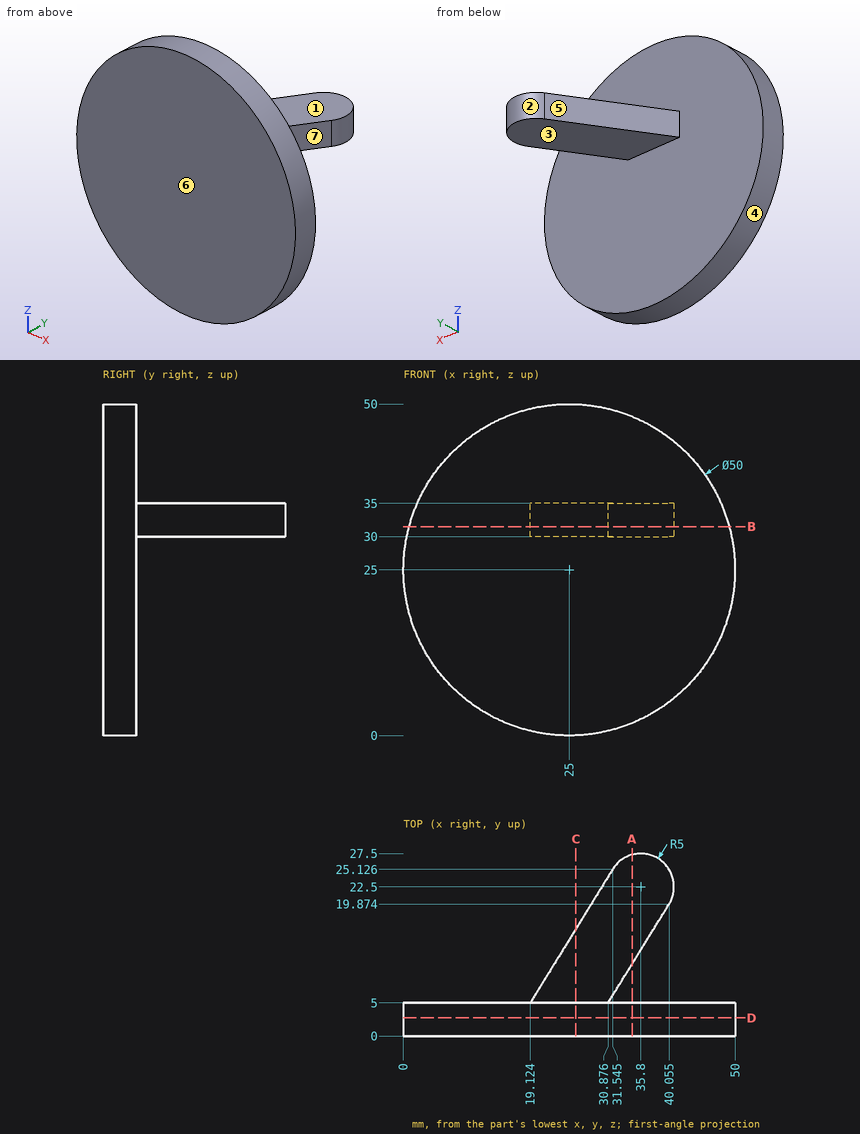
Input: dimensioned drawing with shaded views. Units: mm. Origin: part minimum x, y, z. A direction names the side the tool comes from. Round coordinates to 2 decimals unless told otherwise and drop trailing zeros. Write each loop counter-clockwise with the first axis right and the second up, starting at its lowest first coordinate (ties: lowest second). Pieces come first, ordered by that corner, then holes. Notation, with made-up numbers: (36.5, 32.5) - (92.5, 32.5) arc R12 ccw to (92.5, 41.5) - close; hole circle Ø9 at (6, 76.5). An arc over 180 degrees is marked (long way). Write item = value, one per line.
(1) Section query D-D on y = 2.75. Output: boundary loops of the cut face in (x, z), then the cut area to 3 significant figures.
Geometry check:
outline = circle Ø50 at (25, 25)
area = 1,960 mm^2
(2) Section query A-A on x = 34.5. Output: boundary loops of the cut face in (y, z) (1 decimal).
Geometry check:
outline = (0, 1.9) - (5, 1.9) - (5, 48.1) - (0, 48.1) - close; (10.9, 30) - (27.3, 30) - (27.3, 35) - (10.9, 35) - close
(3) Material intervals for probe 1 along Z at (x, y) = (30.5, 8); probe 2 along Y at (x, z) = (11, 45.5); probe 3 along Y at (x, z) = (33, 31.5) (1 decimal), sorted ascending.
Geometry check:
probe_1 = 30 to 35
probe_2 = 0 to 5
probe_3 = 0 to 5, 8.4 to 26.6
(4) Section query B-B on z = 31.5. Output: boundary loops of the cut face in (x, y) (1 decimal).
Geometry check:
outline = (0.9, 0) - (49.1, 0) - (49.1, 5) - (30.9, 5) - (40.1, 19.9) arc R5 ccw to (31.5, 25.1) - (19.1, 5) - (0.9, 5) - close
(5) Contact query for flat-ended pins moving along their axis: pin 1 Ø2 at (x, y) = (39, 4.5) entering from -Z (1 decimal); pin 2 Ø10 at (y, z) = (5.5, 5) entering from +X; pin 3 Ø3 at (x, z) = (38.5, 34) entering from +Y. Output: stop coordinate, or through.
Geometry check:
pin_1 = 3.6
pin_2 = 44.98
pin_3 = 27.35
(6) Access query for the marked faces 1, 2 and 3. Directions: +Z, -Z, +X, -X, +Y, -Y. A direction counts if a zero-diameter tool reaches every point of the face in a straight line with its end or side. Return the directions, or none.
Geometry check:
face_1 = +Z, +X, -X, +Y
face_2 = +Z, -Z
face_3 = -Z, +X, -X, +Y
(7) Pull-direction query (Y, two-part tool) for the marked faces 4, 5, 6 and 7; classes: +Y half, -Y half, draft (parallel to the pull), parting line (faces both ways), or undercut.
Geometry check:
face_4 = draft
face_5 = +Y half
face_6 = -Y half
face_7 = undercut
(8) Section query C-C on x = 26. Output: boundary loops of the cut face in (y, z).
Geometry check:
outline = (0, 0.02) - (5, 0.02) - (5, 30) - (16.14, 30) - (16.14, 35) - (5, 35) - (5, 49.98) - (0, 49.98) - close
